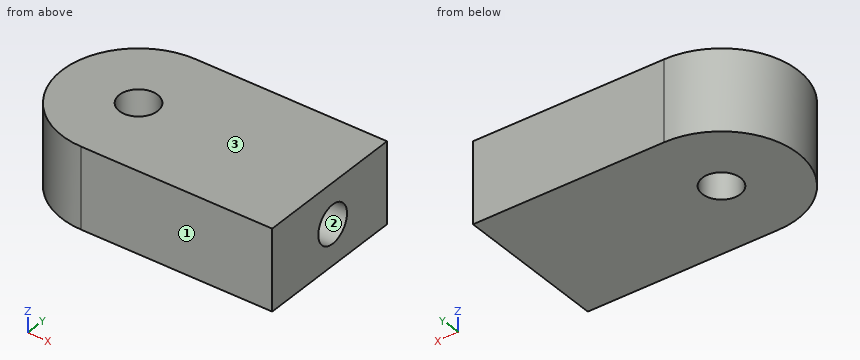
```python
from build123d import *

# Parameters (mm, degrees)
BOSS_EXTRU_1_DEPTH      = 6.35
ESQUISSE3_R             = 1.5
ENL_V_MAT_EXTRU_1_DEPTH = 6.35
ESQUISSE4_R             = 1.5
ENL_V_MAT_EXTRU_2_DEPTH = 6.35


with BuildPart() as part:
    # Esquisse2 → Boss.-Extru.1 (new body)
    with BuildSketch(Plane.XY):
        with BuildLine():
            Line((0, 6), (15, 6))
            Line((15, 6), (15, -6))
            Line((15, -6), (0, -6))
            ThreePointArc((0, -6), (-6, 0), (0, 6))
        make_face()
    extrude(amount=BOSS_EXTRU_1_DEPTH)

    # Esquisse3 → Enlèv. mat.-Extru.1 (cut)
    with BuildSketch(Plane(origin=(15, 0, 0), x_dir=(0, 0, -1), z_dir=(1, 0, 0))):
        with Locations(Location((-3.175, 0.318926735, 0), (0, 0, 90))):
            Circle(ESQUISSE3_R)
    extrude(amount=-ENL_V_MAT_EXTRU_1_DEPTH, mode=Mode.SUBTRACT)

    # Esquisse4 → Enlèv. mat.-Extru.2 (cut)
    with BuildSketch(Plane.XY.offset(6.35)):
        Circle(ESQUISSE4_R)
    extrude(amount=-ENL_V_MAT_EXTRU_2_DEPTH, mode=Mode.SUBTRACT)


solid = part.part
```
The listing builds one solid part. Answer for the finished solid, in the listing's coordinates (mm). Face numbers are marked on the shaded views. Round coordinates to 2 decimals unless told otherwise and drop trailing zeros. Write each loop counter-clockwise with the first axis right and the second up, starting at its lowest first coordinate (ties: lowest second). Pieces come first, ordered by that corner, then holes. Notation, with made-up numbers: (15.25, 30.25) -> (26.25, 30.25) arc R15 ccw to (26.25, 48.25) -> close; hole circle Ø3 at (78, 79.5). An arc over 180 degrees is marked (long way). Answer as a JSON object with one key per item and string values. Group by question number.
Q1. Section A-A (z = 5.5) is taken. Write down the section's boundary in (x, y).
Q2. Section D-D (z = 4.25) is taken. Write down the section's boundary in (x, y), plus the area to 3 significant figures.
Q3. Section B-B (z = 2.75) is taken. Write down the section's boundary in (x, y), plus the area to 3 significant figures.
Q4. Determine the mould class of the marked faces 1, 2 and 3 for opening direction Y: pulls with the +Y half, pulls with the -Y half, needs draft (parallel to the pull), parting line crosses it, or undercut.
Q5. Section C-C (y = 2.25) is taken. Write down the section's boundary in (x, z), plus the area to 3 significant figures.
Q6. Straight lines are drawn through the part: line 1 along Y through (x, z) = (0, 3); line 2 along X through (y, z) = (0.75, 6); line 3 along X through (y, z) = (1, 3). For each, find the intervals that lie inside material, in ascending order.
Check values:
{
 "1": {"outline": "(0, -6) -> (15, -6) -> (15, 6) -> (0, 6) arc R6 ccw to start; hole circle Ø3 at (0, 0)"},
 "2": {"outline": "(0, -6) -> (15, -6) -> (15, -0.73) -> (8.65, -0.73) -> (8.65, 1.37) -> (15, 1.37) -> (15, 6) -> (0, 6) arc R6 ccw to start; hole circle Ø3 at (0, 0)", "area": "216 mm^2"},
 "3": {"outline": "(0, -6) -> (15, -6) -> (15, -1.12) -> (8.65, -1.12) -> (8.65, 1.76) -> (15, 1.76) -> (15, 6) -> (0, 6) arc R6 ccw to start; hole circle Ø3 at (0, 0)", "area": "211 mm^2"},
 "4": {"face 1": "pulls with the -Y half", "face 2": "undercut", "face 3": "needs draft"},
 "5": {"outline": "(-5.56, 0) -> (15, 0) -> (15, 6.35) -> (-5.56, 6.35) -> close", "area": "131 mm^2"},
 "6": {"line 1": "-6 to -1.5, 1.5 to 6", "line 2": "-5.95 to -1.3, 1.3 to 15", "line 3": "-5.92 to -1.12, 1.12 to 8.65"}
}
